```python
from build123d import *

# Parameters (mm, degrees)
F0_W          = 19.812
F0_H          = 76.2
F0_H_2        = 88.9
F0_H_3        = 292.1
F1_DEPTH      = 836.676
F2_DEPTH      = 19.812
F2_DEPTH_BACK = 856.488


with BuildPart() as f1:
    # F0 (on Right) → F1 (new body)
    with BuildSketch(Plane.YZ):
        with Locations((-55.2229133244, 98.4447455046)):
            Rectangle(F0_W, F0_H)
        with Locations((-55.2229133244, 466.7447455046)):
            Rectangle(F0_W, F0_H)
        with Locations((-55.2229133244, 549.2947455046)):
            Rectangle(F0_W, F0_H_2)
        with Locations((-55.2229133244, 282.5947455046)):
            Rectangle(F0_W, F0_H_3)
        with Locations((-55.2229133244, 22.2447455046)):
            Rectangle(F0_W, F0_H)
    extrude(amount=F1_DEPTH)

    # F0 (on Right) → F2 (join, two sides)
    with BuildSketch(Plane.YZ) as f2_sk:
        with Locations((-55.2229133244, 466.7447455046)):
            Rectangle(F0_W, F0_H)
        with Locations((-55.2229133244, 98.4447455046)):
            Rectangle(F0_W, F0_H)
    extrude(amount=-F2_DEPTH)
    extrude(f2_sk.sketch, amount=F2_DEPTH_BACK)


solid = f1.part
```
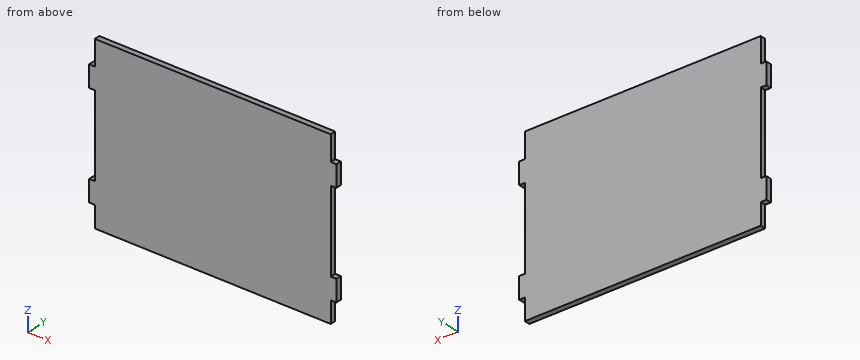
For this review, take the finished solid that the model builds, in its own axes (mm). Round coordinates to 2 decimals unless told otherwise and drop trailing zeros. Write each loop counter-clockwise with the first axis right and the second up, starting at its lowest first coordinate (ties: lowest second). Pieces come first, ordered by that corner, then holes. Notation, with made-up numbers: (73, -28.75) - (86, -28.75) arc R13 cw to (86, -4.75) - close; hole circle Ø7 at (1, 53). An arc over 180 degrees is marked (long way). Put each result on its own line as item: value.
Q1. Wall thickness on probe 1 along X at (y, z) = (-60.5, 243): over which ranges is the line inside the solid? List them lowest first.
Solved:
probe 1: x = 0 to 836.68
Q2. We need section B-B (z = 167). Give the boundary of the cut face in (x, y).
Solved:
outline: (0, -65.13) - (836.68, -65.13) - (836.68, -45.32) - (0, -45.32) - close
Q3. We need section A-A (y = -56.75). Give the boundary of the cut face in (x, z).
Solved:
outline: (-19.81, 60.34) - (0, 60.34) - (0, -15.86) - (836.68, -15.86) - (836.68, 60.34) - (856.49, 60.34) - (856.49, 136.54) - (836.68, 136.54) - (836.68, 428.64) - (856.49, 428.64) - (856.49, 504.84) - (836.68, 504.84) - (836.68, 593.74) - (0, 593.74) - (0, 504.84) - (-19.81, 504.84) - (-19.81, 428.64) - (0, 428.64) - (0, 136.54) - (-19.81, 136.54) - close
Q4. Insertion check: pin 1 Ø10 at (x, y) = (849, -50.5) entering from -Z; pin 2 Ø10 at (x, y) = (847.5, -50.5) entering from +Z; pin 3 Ø3 at (y, z) = (-52.5, 246) entering from -X. Each pin has a flat end and moves straight along its axis. Give the tip position at first contact, or say it passes through.
Solved:
pin 1: stops at z = 60.34
pin 2: stops at z = 504.84
pin 3: stops at x = 0
